from build123d import *

# Parameters (mm, degrees)
SKETCH1_R           = 32.5
SKETCH1_R_2         = 9.5
SKETCH1_R_3         = 3.1
BOSS_EXTRUDE1_DEPTH = 4
SKETCH2_R           = 12.5
SKETCH2_R_2         = 9.5
BOSS_EXTRUDE2_DEPTH = 200
SKETCH3_R           = 32.5
SKETCH3_R_2         = 3.1
SKETCH3_R_3         = 9.5
BOSS_EXTRUDE3_DEPTH = 4


with BuildPart() as part:
    # Sketch1 → Boss-Extrude1 (new body)
    with BuildSketch(Plane(origin=(0, 0, 0), x_dir=(1, 0, 0), z_dir=(0, 1, 0))):
        with Locations(Location((0, 0, 0), (0, 0, 270))):
            Circle(SKETCH1_R)
        with Locations(Location((0, 0, 0), (0, 0, 270))):
            Circle(SKETCH1_R_2, mode=Mode.SUBTRACT)
        with Locations(Location((-17.5, 17.5, 0), (0, 0, 270))):
            Circle(SKETCH1_R_3, mode=Mode.SUBTRACT)
        with Locations(Location((17.5, 17.5, 0), (0, 0, 270))):
            Circle(SKETCH1_R_3, mode=Mode.SUBTRACT)
        with Locations(Location((17.5, -17.5, 0), (0, 0, 270))):
            Circle(SKETCH1_R_3, mode=Mode.SUBTRACT)
        with Locations(Location((-17.5, -17.5, 0), (0, 0, 270))):
            Circle(SKETCH1_R_3, mode=Mode.SUBTRACT)
    extrude(amount=BOSS_EXTRUDE1_DEPTH)

    # Sketch2 → Boss-Extrude2 (add)
    with BuildSketch(Plane(origin=(0, 4, 0), x_dir=(1, 0, 0), z_dir=(0, 1, 0))):
        with Locations(Location((0, 0, 0), (0, 0, 270))):
            Circle(SKETCH2_R)
        with Locations(Location((0, 0, 0), (0, 0, 270))):
            Circle(SKETCH2_R_2, mode=Mode.SUBTRACT)
    extrude(amount=BOSS_EXTRUDE2_DEPTH)

    # Sketch3 → Boss-Extrude3 (add)
    with BuildSketch(Plane(origin=(0, 204, 0), x_dir=(1, 0, 0), z_dir=(0, 1, 0))):
        with Locations(Location((0, 0, 0), (0, 0, 270))):
            Circle(SKETCH3_R)
        with Locations(Location((-17.5, 17.5, 0), (0, 0, 270))):
            Circle(SKETCH3_R_2, mode=Mode.SUBTRACT)
        with Locations(Location((17.5, 17.5, 0), (0, 0, 270))):
            Circle(SKETCH3_R_2, mode=Mode.SUBTRACT)
        with Locations(Location((17.5, -17.5, 0), (0, 0, 270))):
            Circle(SKETCH3_R_2, mode=Mode.SUBTRACT)
        with Locations(Location((-17.5, -17.5, 0), (0, 0, 270))):
            Circle(SKETCH3_R_2, mode=Mode.SUBTRACT)
        with Locations(Location((0, 0, 0), (0, 0, 270))):
            Circle(SKETCH3_R_3, mode=Mode.SUBTRACT)
    extrude(amount=BOSS_EXTRUDE3_DEPTH)


solid = part.part
Geometry check sheet. Reference: the model listing, model coordinates, mm. A direction names the side the tool comes from. Give positions to 0.01 mm unless a question says otherwise; leave off trailing zeros. Loops run counter-clockwise (first coordinate to the right, second up) from the corner with the lowest first, then second, coordinate; pieces in that order, holes last. Notation, with made-up numbers: (56, -37) -> (64, -37) arc R22 ccw to (64, -24) -> close; hole circle Ø10 at (21, 32). An arc over 180 degrees is marked (long way). Answer in a Markdown table with one row per item. Add a question column.
1) Cross-section at A-A on z = 0. Record the boundary of the cut face in (x, y), and give its area (3 significant figures).
2) Draft check along Z on faces 3 (the face through (15.614, 205.972, -19.96)), 4 (the face through (-7, 208, 7)), 5 (the face through (9.76, 205.97, 31)). Enter one of: pulls with the +Z half, pulls with the -Z half, needs draft (parallel to the pull), parting line crosses it, or undercut.
3) Gauge pin test, flat ends, axial feed: P1, Ø8, axis at y = 93.5, z = -15.5, coming from the +X side; P2, Ø5, axis at x = 17.5, z = 17.5, coming from the -Y side; P3, Ø10, axis at y = 175.5, z = 13.5, coming from the -X side; P4, Ø8, axis at x = 10.5, y = 93.5, coming from the +Z side. Record the tip position at first contact, or that the pin passes through.
4) Set-up check for faces 1 (the face through (-5.78, 102.54, -7.54)), 2 (the face through (0, 204, 14)): record each of +Z, -Z, +X, -X, +Y, -Y from which the full face is reachable in a straight line by a thin tool's end or side.
5) Cross-section at C-C on z = 18.5. Record the boundary of the cut face in (x, y).
6) Material ranges on probe 1 along Y at (x, z) = (-22, 17); probe 2 along X at (y, z) = (1.8, 17.5); probe 3 along X at (y, z) = (206, -17), recorded low to high. Write a range as from..to.
7) Cross-section at B-B on x = 0. Record the boundary of the cut face in (y, z).
8) Cross-section at D-D on y = 77. Record the boundary of the cut face in (x, z), and give its area (3 significant figures).
Outcome:
| question | item | result |
|---|---|---|
| 1 | outline | (-32.5, 0) -> (-9.5, 0) -> (-9.5, 208) -> (-32.5, 208) -> (-32.5, 204) -> (-12.5, 204) -> (-12.5, 4) -> (-32.5, 4) -> close; (9.5, 0) -> (32.5, 0) -> (32.5, 4) -> (12.5, 4) -> (12.5, 204) -> (32.5, 204) -> (32.5, 208) -> (9.5, 208) -> close |
| 1 | area | 1,570 mm^2 |
| 2 | face 3 | undercut |
| 2 | face 4 | needs draft |
| 2 | face 5 | parting line crosses it |
| 3 | P1 | stops at x = 4.9 |
| 3 | P2 | passes through |
| 3 | P3 | stops at x = -9.17 |
| 3 | P4 | stops at z = 10.68 |
| 4 | face 1 | +Y, -Y |
| 4 | face 2 | none |
| 5 | outline | (-26.72, 0) -> (-20.43, 0) -> (-20.43, 4) -> (-26.72, 4) -> close; (-26.72, 204) -> (-20.43, 204) -> (-20.43, 208) -> (-26.72, 208) -> close; (-14.57, 0) -> (14.57, 0) -> (14.57, 4) -> (-14.57, 4) -> close; (-14.57, 204) -> (14.57, 204) -> (14.57, 208) -> (-14.57, 208) -> close; (20.43, 0) -> (26.72, 0) -> (26.72, 4) -> (20.43, 4) -> close; (20.43, 204) -> (26.72, 204) -> (26.72, 208) -> (20.43, 208) -> close |
| 6 | probe 1 | y = 0..4, 204..208 |
| 6 | probe 2 | x = -27.39..-20.6, -14.4..14.4, 20.6..27.39 |
| 6 | probe 3 | x = -27.7..-20.56, -14.44..14.44, 20.56..27.7 |
| 7 | outline | (0, -32.5) -> (4, -32.5) -> (4, -12.5) -> (204, -12.5) -> (204, -32.5) -> (208, -32.5) -> (208, -9.5) -> (0, -9.5) -> close; (0, 9.5) -> (208, 9.5) -> (208, 32.5) -> (204, 32.5) -> (204, 12.5) -> (4, 12.5) -> (4, 32.5) -> (0, 32.5) -> close |
| 8 | outline | circle Ø25 at (0, 0); hole circle Ø19 at (0, 0) |
| 8 | area | 207 mm^2 |
